Check sheet for the modelled part. Datum: model origin and axes. Units: mm. Round coordinates to 2 decimals unless told otherwise and drop trailing zeros.
Item 1: Section check A-A, the plane z = 1. State how many separate pieces and enclosed holes the cut face has, plus the area to 3 significant figures.
Item 2: Material ranges on line 1 along X through (y, z) = (2680.75, 0.9); line 2 along Y through (x, z) = (6557, 0.9), recorded low to high.
Item 3: Depth check by flat-ended pin: pin 1 (0.5 mm diameter, centred on y = 2683, z = 1, fed in from +X); pin 2 (0.8 mm diameter, centred on y = 2683.5, z = 0.5, fed in from -X). Enter the tip coordinate at first touch or a pass-through.
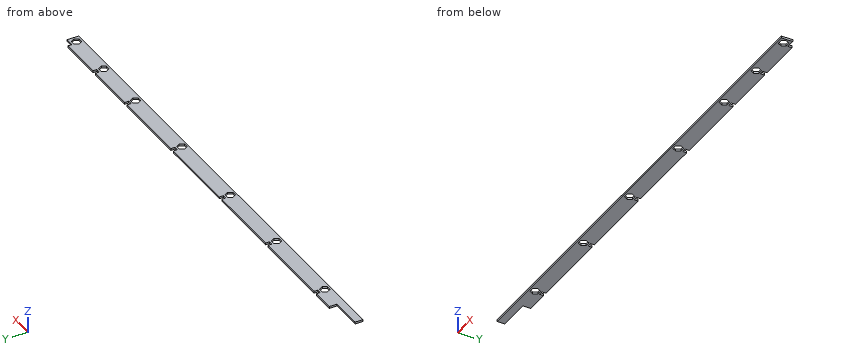
from build123d import *

# Parameters (mm, degrees)
BOSS_EXTRUDE1_DEPTH = 1.5875


with BuildPart() as part:
    # Sketch1 → Boss-Extrude1 (new body)
    with BuildSketch(Plane.XY):
        Polygon((6838.872739, 2682.026941165), (6838.872739, 2685.201941165), (6803.727441916, 2685.201941165), (6803.727441916, 2682.026941165), (6800.323841916, 2682.026941165), (6800.323841916, 2685.201941165), (6759.161189, 2685.201941165), (6759.161189, 2682.026941165), (6755.757589, 2682.026941165), (6755.757589, 2685.201941165), (6694.276889, 2685.201941165), (6694.276889, 2682.026941165), (6690.873289, 2682.026941165), (6690.873289, 2685.201941165), (6626.217589, 2685.201941165), (6626.217589, 2682.026941165), (6622.813989, 2682.026941165), (6622.813989, 2685.201941165), (6561.333289, 2685.201941165), (6561.333289, 2682.026941165), (6557.929689, 2682.026941165), (6557.929689, 2685.201941165), (6493.273989, 2685.201941165), (6493.273989, 2682.026941165), (6489.870389, 2682.026941165), (6489.870389, 2685.201941165), (6471.830039, 2685.201941165), (6471.830039, 2679.017041165), (6446.430039, 2679.017041165), (6446.430039, 2672.832141165), (6845.679939, 2672.832141165), (6845.679939, 2682.026941165), align=None)
        Polygon((6493.519576105, 2674.254541165), (6495.35266321, 2677.429541165), (6493.519576105, 2680.604541165), (6489.853401896, 2680.604541165), (6488.020314791, 2677.429541165), (6489.853401896, 2674.254541165), align=None, mode=Mode.SUBTRACT)
        Polygon((6561.578876105, 2674.254541165), (6563.41196321, 2677.429541165), (6561.578876105, 2680.604541165), (6557.912701896, 2680.604541165), (6556.079614791, 2677.429541165), (6557.912701896, 2674.254541165), align=None, mode=Mode.SUBTRACT)
        Polygon((6626.463176105, 2674.254541165), (6628.29626321, 2677.429541165), (6626.463176105, 2680.604541165), (6622.797001896, 2680.604541165), (6620.963914791, 2677.429541165), (6622.797001896, 2674.254541165), align=None, mode=Mode.SUBTRACT)
        Polygon((6694.522476105, 2674.254541165), (6696.35556321, 2677.429541165), (6694.522476105, 2680.604541165), (6690.856301896, 2680.604541165), (6689.023214791, 2677.429541165), (6690.856301896, 2674.254541165), align=None, mode=Mode.SUBTRACT)
        Polygon((6759.406776105, 2674.254541165), (6761.23986321, 2677.429541165), (6759.406776105, 2680.604541165), (6755.740601896, 2680.604541165), (6753.907514791, 2677.429541165), (6755.740601896, 2674.254541165), align=None, mode=Mode.SUBTRACT)
        Polygon((6803.973029021, 2674.254541165), (6805.806116126, 2677.429541165), (6803.973029021, 2680.604541165), (6800.306854812, 2680.604541165), (6798.473767707, 2677.429541165), (6800.306854812, 2674.254541165), align=None, mode=Mode.SUBTRACT)
        Polygon((6842.521926105, 2674.254541165), (6844.35501321, 2677.429541165), (6842.521926105, 2680.604541165), (6838.855751896, 2680.604541165), (6837.022664791, 2677.429541165), (6838.855751896, 2674.254541165), align=None, mode=Mode.SUBTRACT)
    extrude(amount=BOSS_EXTRUDE1_DEPTH)


solid = part.part
Values found:
1. separate pieces: 1
1. enclosed holes: 7
1. area: 4,450 mm2
2. line 1: x = 6471.83 to 6845.68
2. line 2: y = 2672.83 to 2675.84, 2679.02 to 2685.2
3. pin 1: stops at x = 6838.87
3. pin 2: stops at x = 6471.83
